Could you check a few things on this model? Use its own coordinates, in mm. Face numbers are marked on the shaded views. A direction names the side the tool comes from. Round coordinates to 2 decimals unless told otherwise and drop trailing zeros. Write each loop counter-clockwise with the first axis right and the second up, starting at its lowest first coordinate (ties: lowest second). Pieces come first, ordered by that corner, then holes. Notation, with made-up numbers: M 85,-39 L 91,-39 A5 ccw 91,-32 Z; hole C -14.75,67 d2. An arc over 180 degrees is marked long. One line per question, with ' | ' between items. Start each with the question number.
```python
from build123d import *

# Parameters (mm, degrees)
SKETCH1_W           = 7.9
SKETCH1_H           = 7.9
BOSS_EXTRUDE1_DEPTH = 9.6
CUT_EXTRUDE1_DEPTH  = 9.6
SKETCH3_R           = 2.8
CUT_EXTRUDE2_DEPTH  = 0.5
CUT_EXTRUDE3_START  = -0.5
SKETCH4_R           = 2.8
SKETCH4_R_2         = 2.4
CUT_EXTRUDE3_DEPTH  = 0.5
SKETCH5_R           = 2.4
BOSS_EXTRUDE2_DEPTH = 1.7
CUT_EXTRUDE4_DEPTH  = 1.7


with BuildPart() as part:
    # Sketch1 → Boss-Extrude1 (new body)
    with BuildSketch(Plane(origin=(0, 0, 0), x_dir=(1, 0, 0), z_dir=(0, 1, 0))):
        with Locations((3.95, 3.95)):
            Rectangle(SKETCH1_W, SKETCH1_H)
    extrude(amount=BOSS_EXTRUDE1_DEPTH)

    # Sketch2 → Cut-Extrude1 (cut)
    with BuildSketch(Plane.XY):
        with BuildLine():
            ThreePointArc((3.95, 7.999162379), (1.55, 5.599162379), (3.95, 3.199162379))
            Line((3.95, 3.199162379), (3.95, 3.2))
            Line((3.95, 3.2), (3.95, 7.998324758))
            Line((3.95, 7.998324758), (3.95, 7.999162379))
        make_face()
        with BuildLine():
            Line((3.95, 3.2), (3.95, 3.199162379))
            ThreePointArc((3.95, 3.199162379), (5.647056275, 3.902106104), (6.35, 5.599162379))
            ThreePointArc((6.35, 5.599162379), (5.647056275, 7.296218654), (3.95, 7.999162379))
            Line((3.95, 7.999162379), (3.95, 7.998324758))
            Line((3.95, 7.998324758), (3.95, 3.2))
        make_face()
    extrude(amount=-CUT_EXTRUDE1_DEPTH, mode=Mode.SUBTRACT)

    # Sketch3 → Cut-Extrude2 (cut)
    with BuildSketch(Plane.XY):
        with Locations((3.95, 5.599162379)):
            Circle(SKETCH3_R)
    extrude(amount=-CUT_EXTRUDE2_DEPTH, mode=Mode.SUBTRACT)

    # Sketch4 → Cut-Extrude3 (cut)
    with BuildSketch(Plane(origin=(0, 0, -7.9), x_dir=(-1, 0, 0), z_dir=(0, 0, -1)).offset(CUT_EXTRUDE3_START)):
        with Locations(Location((-3.95, 5.599162379, 0), (0, 0, 180))):
            Circle(SKETCH4_R)
        with Locations(Location((-3.95, 5.599162379, 0), (0, 0, 180))):
            Circle(SKETCH4_R_2, mode=Mode.SUBTRACT)
    extrude(amount=CUT_EXTRUDE3_DEPTH, mode=Mode.SUBTRACT)

    # Sketch5 → Boss-Extrude2 (add)
    with BuildSketch(Plane(origin=(0, 9.6, 0), x_dir=(1, 0, 0), z_dir=(0, 1, 0))):
        with Locations(Location((3.95, 3.95, 0), (0, 0, 270))):
            Circle(SKETCH5_R)
    extrude(amount=BOSS_EXTRUDE2_DEPTH)

    # Sketch6 → Cut-Extrude4 (cut)
    with BuildSketch(Plane(origin=(0, 11.3, 0), x_dir=(1, 0, 0), z_dir=(0, 1, 0))):
        with BuildLine():
            ThreePointArc((5.65, 3.95), (3.95, 5.65), (2.25, 3.95))
            Line((2.25, 3.95), (5.65, 3.95))
        make_face()
        with BuildLine():
            Line((5.65, 3.95), (2.25, 3.95))
            ThreePointArc((2.25, 3.95), (3.95, 2.25), (5.65, 3.95))
        make_face()
    extrude(amount=-CUT_EXTRUDE4_DEPTH, mode=Mode.SUBTRACT)

    # Mirror1: part across plane


with BuildPart() as part_1:
    add(part.part)
    add(part.part.mirror(Plane(origin=(7.9, 9.6, 0), x_dir=(0, 0, 1), z_dir=(-1, 0, 0))))


solid = part_1.part
```
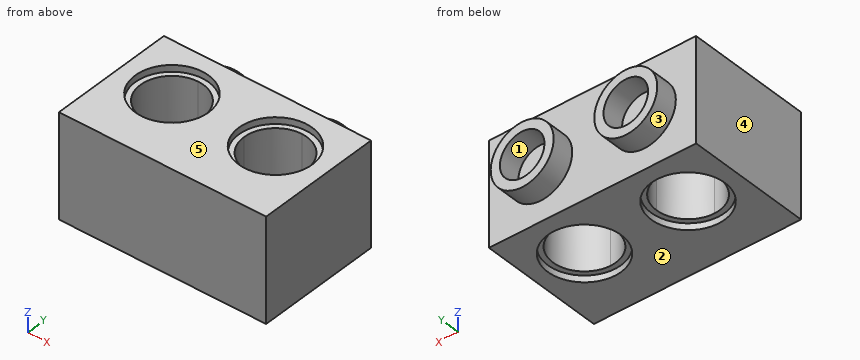
1. Suppose I cut it at C-C (y = 7). Write out the boundary of the cut face in (x, z), and give its area (3 significant figures).
2. Which directions (+Z, -Z, +X, -X, +Y, -Y) give clear straight access to the entire face, cutting with the end or side of a thin tool? Please do the marked faces 1 and 2.
3. If we mould it in two halves opening along X, with no side actions, what happens to the marked faces 3, 4 and 5? For each: released by +X, released by -X, zero draft, split by the parting line, or undercut.
4. Suppose I cut it at B-B (x = 12.75). Write out the boundary of the cut face in (y, z), and give its area (3 significant figures).
5. I'm going to push flat-ended pins straight in: P1, Ø2, axis at x = 2.5, y = 5, coming from the -Z side; P2, Ø3, axis at x = 13.5, y = 8.5, coming from the +Z side; P3, Ø1.7, axis at x = 12, z = -4.5, coming from the +Y side; P4, Ø3, axis at x = 3, y = 5, coming from the +Z side. Where does each tip first touch, or does it pass through?
6. Suppose I cut it at D-D (z = -3.95). Write out the boundary of the cut face in (x, y).
7. Suppose I cut it at A-A (z = -6.75). Write out the boundary of the cut face in (x, y).
8. I need wall thicknesses on line 1 along X through (y, z) = (5.5, -2.5); line 2 along Y through (x, z) = (3.95, -0.25); line 3 along X through (y, z) = (7.25, -4). Which ranges of each line are inside material? Lowest first, please. Write a range as from..to.
Computed:
1) outline: M 0,-7.9 L 1.53,-7.9 L 1.53,-7.4 L 2,-7.4 L 2,-0.5 L 1.53,-0.5 L 1.53,0 L 0,0 Z; M 5.9,-7.4 L 6.37,-7.4 L 6.37,-7.9 L 9.43,-7.9 L 9.43,-7.4 L 9.9,-7.4 L 9.9,-0.5 L 9.43,-0.5 L 9.43,0 L 6.37,0 L 6.37,-0.5 L 5.9,-0.5 Z; M 13.8,-7.4 L 14.27,-7.4 L 14.27,-7.9 L 15.8,-7.9 L 15.8,0 L 14.27,0 L 14.27,-0.5 L 13.8,-0.5 Z | area: 61.3 mm²
2) face 1: +Y | face 2: -Z, +X, -X, +Y, -Y
3) face 3: undercut | face 4: released by -X | face 5: zero draft
4) outline: M 0,-7.9 L 2.95,-7.9 L 2.95,-7.4 L 3.37,-7.4 L 3.37,-0.5 L 2.95,-0.5 L 2.95,0 L 0,0 Z; M 7.82,-7.4 L 8.25,-7.4 L 8.25,-7.9 L 9.6,-7.9 L 9.6,-6.17 L 11.3,-6.17 L 11.3,-5.39 L 9.6,-5.39 L 9.6,-2.51 L 11.3,-2.51 L 11.3,-1.73 L 9.6,-1.73 L 9.6,0 L 8.25,0 L 8.25,-0.5 L 7.82,-0.5 Z | area: 42.5 mm²
5) P1: stops at z = -7.4 | P2: stops at z = 0 | P3: stops at y = 9.6 | P4: stops at z = -0.5
6) outline: M 0,0 L 15.8,0 L 15.8,9.6 L 14.25,9.6 L 14.25,11.3 L 13.55,11.3 L 13.55,9.6 L 10.15,9.6 L 10.15,11.3 L 9.45,11.3 L 9.45,9.6 L 6.35,9.6 L 6.35,11.3 L 5.65,11.3 L 5.65,9.6 L 2.25,9.6 L 2.25,11.3 L 1.55,11.3 L 1.55,9.6 L 0,9.6 Z; hole C 3.95,5.6 d4.8; hole C 11.85,5.6 d4.8
7) outline: M 0,0 L 15.8,0 L 15.8,9.6 L 0,9.6 Z; hole C 3.95,5.6 d4.8; hole C 11.85,5.6 d4.8
8) line 1: x = 0..1.55, 6.35..9.45, 14.25..15.8 | line 2: y = 0..2.8, 8.4..9.6 | line 3: x = 0..2.21, 5.69..10.11, 13.59..15.8
